Study the drawing (mm; zero at the part's minimum x, y, z) and answer. A direction names the side the tool comes from. Coordinates: 2 decimals unless noted, no trailing zeros. Loops run counter-clockwise (first coordinate to the right, second up) from the corner with the lowest first, then second, coordinate; pieces in that order, holes last. Notation, with made-up numbers: (60, 18.25) -> (65, 18.25) arc R27 cw to (65, 35.25) -> close; hole circle Ø4 at (16, 6). An arc over 180 degrees is marked (long way). Answer as a JSON object with one key per item and string values. Group by question number.
Q1. For the marked faces 1 and 2, determine the directions among +Z, -Z, +X, -X, +Y, -Y from which every point of the face is accessible in a straight line to the end or side of a thin tool.
Q2. Each of these flat-tipped pins is pushed along its axis until it touches: P1, Ø4, axis at x = 4, y = 19.5, coming from the -Z side; P2, Ø3, axis at y = 4.5, z = 5.5, coming from the +X side. Where does it stop, or does it pass through?
Q3. Straight lines are drawn through the part: line 1 along X through (y, z) = (25, 1.5); line 2 along Z through (x, y) = (35.5, 15); line 3 along Y through (x, z) = (35.5, 5.5). For each, find the intervals that lie inside material, in ascending order. Write a range as [from, to].
Q4. The part is cut by section B-B on y = 14. Write down the section's boundary in (x, z), and give its area (3 significant figures).
Q5. The part is cut by section A-A on z = 6.65. Write down the section's boundary in (x, y), and give its area (3 significant figures).
Q6. The part is cut by section C-C on x = 32.5. Write down the section's boundary in (y, z), and give its area (3 significant figures).
Q7. The part is cut by section D-D on z = 1. Write down the section's boundary in (x, y), and give its area (3 significant figures).
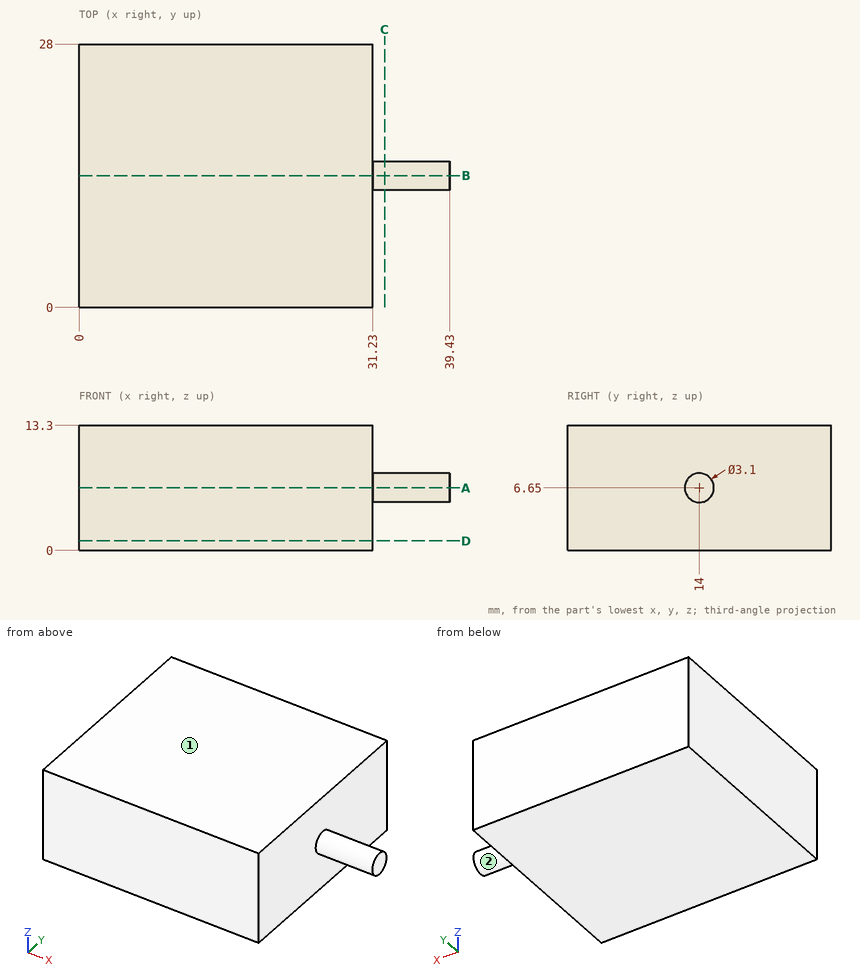
Final values:
{
 "1": {"face 1": "+Z, +X, -X, +Y, -Y", "face 2": "+X"},
 "2": {"P1": "stops at z = 0", "P2": "stops at x = 31.23"},
 "3": {"line 1": "x = [0, 31.23]", "line 2": "z = [5.47, 7.83]", "line 3": "y = [12.96, 15.04]"},
 "4": {"outline": "(0, 0) -> (31.23, 0) -> (31.23, 5.1) -> (39.43, 5.1) -> (39.43, 8.2) -> (31.23, 8.2) -> (31.23, 13.3) -> (0, 13.3) -> close", "area": "441 mm2"},
 "5": {"outline": "(0, 0) -> (31.23, 0) -> (31.23, 12.45) -> (39.43, 12.45) -> (39.43, 15.55) -> (31.23, 15.55) -> (31.23, 28) -> (0, 28) -> close", "area": "900 mm2"},
 "6": {"outline": "circle Ø3.1 at (14, 6.65)", "area": "7.55 mm2"},
 "7": {"outline": "(0, 0) -> (31.23, 0) -> (31.23, 28) -> (0, 28) -> close", "area": "874 mm2"}
}
